For this review, take the finished solid that the model builds, in its own axes (mm). Give positions to 0.01 mm unless a question says otherwise; leave off trailing zeros. Write each loop counter-clockwise with the first axis right and the second up, starting at its lowest first coordinate (ties: lowest second). Pieces come first, ordered by that corner, then holes. Notation, with made-up numbers: (15.5, 37) -> (47.5, 37) arc R10 ccw to (47.5, 56) -> close; hole circle Ø4 at (75, 85.25). An arc over 180 degrees is marked (long way). Return JSON: item names as keys, results as strings.
from build123d import *

# Parameters (mm, degrees)
F0_W     = 156
F0_H     = 70
F0_R     = 15
F1_DEPTH = 18
F3_DEPTH = 156


with BuildPart() as f1:
    # F0 (on Top) → F1 (new body)
    with BuildSketch(Plane.XY):
        with Locations((78, -35)):
            Rectangle(F0_W, F0_H)
        with Locations((78, -35)):
            Circle(F0_R, mode=Mode.SUBTRACT)
    extrude(amount=F1_DEPTH)

    # F2 (on Right) → F3 (cut)
    with BuildSketch(Plane.YZ):
        Polygon((-70, 18), (-70, 0), (-62.531915, 18), align=None)
    extrude(amount=F3_DEPTH, mode=Mode.SUBTRACT)


solid = f1.part
1. For pin 1 (2 mm diameter, centred on x = 138.5, z = 2.5, fed in from +Y), flat-tipped, find the tip position at first contact; note if it passes through.
Results found:
{"pin 1": "stops at y = 0"}
2. Add section C-C, the plane z = 16. State the section outline as (x, y) points.
Results found:
{"outline": "(0, -63.36) -> (156, -63.36) -> (156, 0) -> (0, 0) -> close; hole circle Ø30 at (78, -35)"}
3. Add section D-D, the plane x = 96.5. State the section outline as (y, z) points.
Results found:
{"outline": "(-70, 0) -> (0, 0) -> (0, 18) -> (-62.53, 18) -> close"}
4. Add section B-B, the plane y = -35. State the section outline as (x, z) points.
Results found:
{"outline": "(0, 0) -> (63, 0) -> (63, 18) -> (0, 18) -> close; (93, 0) -> (156, 0) -> (156, 18) -> (93, 18) -> close"}
5. To check wall thickness, follow probe 1 along Y at (x, z) = (78, 7.5); probe 2 along X at (y, z) = (-46, 13.75); probe 3 along Y at (x, z) = (78, 3.5). State the ranges of each line that lie inside material, in increasing order.
Results found:
{"probe 1": "y = -66.89 to -50, -20 to 0", "probe 2": "x = 0 to 67.8, 88.2 to 156", "probe 3": "y = -68.55 to -50, -20 to 0"}
6. The part is to be moulded in two halves that separate along X. For faces 1 (the flat face through (77, -17, 18)), 2 (the cylindrical face through (66.944, -24.862, 8.874)), 3 (the flat face through (156, -35, 9)), say which applies: +X half, -X half, draft (parallel to the pull), parting line (faces both ways), or undercut.
Results found:
{"face 1": "draft", "face 2": "undercut", "face 3": "+X half"}
7. Add section A-A, the plane x = 78. State the section outline as (y, z) points.
Results found:
{"outline": "(-70, 0) -> (-50, 0) -> (-50, 18) -> (-62.53, 18) -> close; (-20, 0) -> (0, 0) -> (0, 18) -> (-20, 18) -> close"}
